Part print with two shaded views. Sizes in mm from the minimum x, y, z corner. A direction names the side the tool comes from. Round coordinates to 2 decimals unless told otherwise and drop trailing zeros. Write each loop counter-clockwise with the first axis right and the second up, starting at its lowest first coordinate (ties: lowest second). Pieces come first, ordered by that corner, then holes. Notation, with made-up numbers: (77, 34.25) - (92, 34.25) arc R16 ccw to (92, 38.25) - close; hole circle Ø4 at (84, -21.5). An arc over 180 degrees is marked (long way). Answer as a JSON object with one key per item and string values. Group by question number.
Item 1: Slice it at D-D, the plane z = 54.5. List the corners of the cut face in (x, y) (1 decimal), then the cut area to 3 significant figures.
Item 2: Slice it at A-A, the plane z = 33. List the corners of the cut face in (x, y) (1 decimal), then the cut area to 3 significant figures.
Item 3: Slice it at C-C, the plane y = 73. List the corners of the cut face in (x, z) (1 decimal), then the cut area to 3 significant figures.
Item 4: Probe line 1 (X direction, y = 73, z = 44) (1 decimal); line 2 (Z direction, x = 81, y = 133.5) (1 decimal); line 3 (Y direction, x = 15.5, z = 26.5). List the from-to ranges inside material, lowest first. Write a range as from..to.
Item 5: Which spindle directions (+Z, -Z, +X, -X, +Y, -Y) get a long thin tool onto all of the face, cutting with end or side? Do the marked faces 1, 2, 3, 4 and 5. Say none if no direction does.
Item 6: Flat gauge pins, fed straight in: pin 1 (1.5 mm diameter, centred on x = 25, y = 125, fed in from -Z); pin 2 (2 mm diameter, centred on y = 137, z = 50, fed in from -X); pin 3 (6 mm diameter, centred on y = 65.5, z = 42.5, fed in from +X). Where does each tip first touch, or does it go through?
Item 7: Slice it at B-B, the plane x = 36. List the corners of the cut face in (y, z) (1 decimal).
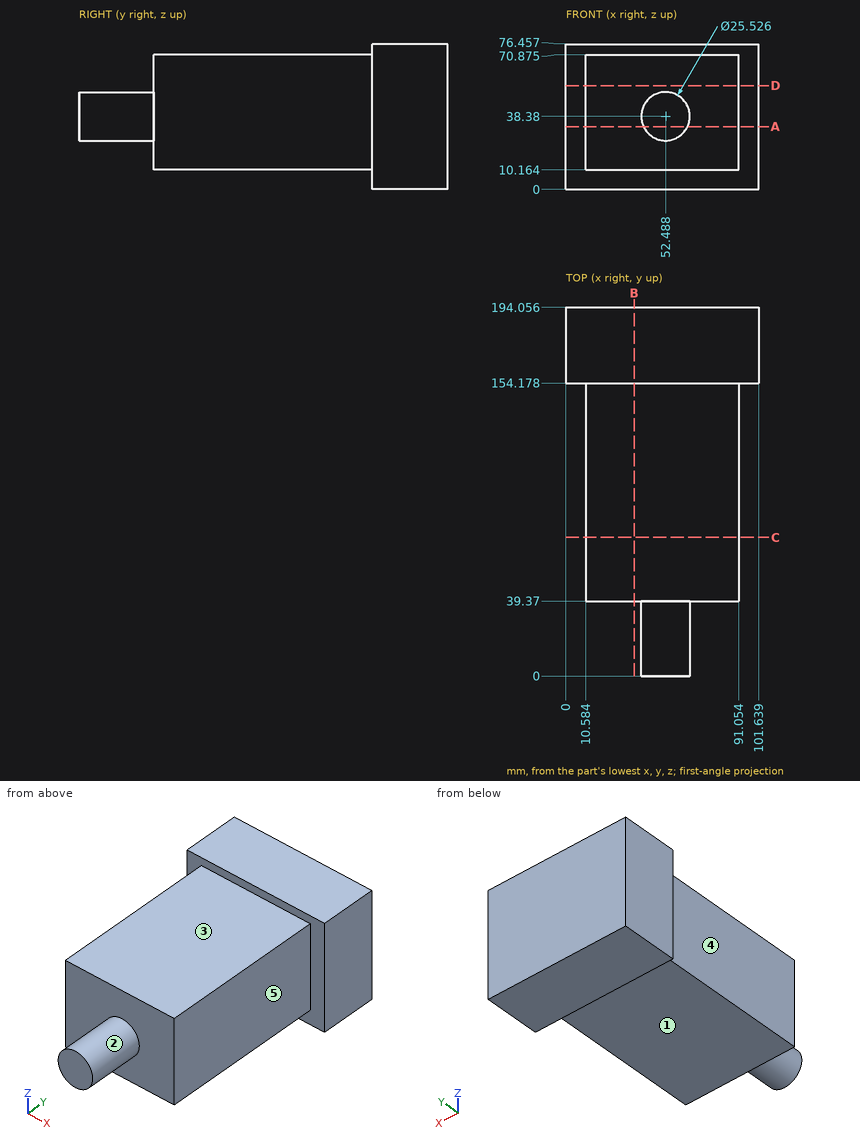
Geometry says:
{
 "1": {"outline": "(0, 154.2) - (10.6, 154.2) - (10.6, 39.4) - (91.1, 39.4) - (91.1, 154.2) - (101.6, 154.2) - (101.6, 194.1) - (0, 194.1) - close", "area": "13,300 mm^2"},
 "2": {"outline": "(0, 154.2) - (10.6, 154.2) - (10.6, 39.4) - (40.9, 39.4) - (40.9, 0) - (64.1, 0) - (64.1, 39.4) - (91.1, 39.4) - (91.1, 154.2) - (101.6, 154.2) - (101.6, 194.1) - (0, 194.1) - close", "area": "14,200 mm^2"},
 "3": {"outline": "(10.6, 10.2) - (91.1, 10.2) - (91.1, 70.9) - (10.6, 70.9) - close", "area": "4,890 mm^2"},
 "4": {"line 1": "x = 10.6..91.1", "line 2": "z = 10.2..70.9", "line 3": "y = 39.37..194.06"},
 "5": {"face 1": "-Z, +X, -X, -Y", "face 2": "-Y", "face 3": "+Z, +X, -X, -Y", "face 4": "+Z, -Z, -X, -Y", "face 5": "+Z, -Z, +X, -Y"},
 "6": {"pin 1": "stops at z = 10.16", "pin 2": "stops at x = 10.58", "pin 3": "stops at x = 91.05"},
 "7": {"outline": "(39.4, 10.2) - (154.2, 10.2) - (154.2, 0) - (194.1, 0) - (194.1, 76.5) - (154.2, 76.5) - (154.2, 70.9) - (39.4, 70.9) - close"}
}
